```python
from build123d import *

# Parameters (mm, degrees)
F0_W     = 38.1
F0_H     = 38.1
F0_W_2   = 31.75
F0_H_2   = 31.75
F1_DEPTH = 2743.2
F2_R     = 6.35
F3_DEPTH = 38.101


# Not quite as in the source:
# - a feature names something its author has since deleted; it is built from what else it names


with BuildPart() as f1:
    # F0 (on Front) → F1 (new body)
    with BuildSketch(Plane.XZ):
        Rectangle(F0_W, F0_H)
        Rectangle(F0_W_2, F0_H_2, mode=Mode.SUBTRACT)
    extrude(amount=F1_DEPTH)

    # F2 (on face) → F3 (cut, through all)
    with BuildSketch(Plane.XY.offset(19.05)):
        with Locations((0, -25.4)):
            Circle(F2_R)
        with Locations((0, -76.2)):
            Circle(F2_R)
        with Locations((0, -2717.8)):
            Circle(F2_R)
        with Locations((0, -2667)):
            Circle(F2_R)
    extrude(amount=-F3_DEPTH, mode=Mode.SUBTRACT)


solid = f1.part
```
Check sheet for the modelled part. Datum: model origin and axes. Units: mm. Round coordinates to 2 decimals unless told otherwise and drop trailing zeros. Loops run counter-clockwise (first coordinate to the right, second up) from the corner with the lowest first, then second, coordinate; pieces in that order, holes last. Notation, with made-up numbers: (24.5, 19.25) -> (63.5, 19.25) arc R18 ccw to (63.5, 51.25) -> close; hole circle Ø2 at (75.25, -27.5). An arc over 180 degrees is marked (long way). Answer in a Markdown table with one row per item.
Q1. Sectioned sample at A-A on z = 6. Enter the section's corners in (x, y) (3 decimals), then the cut area to 3 significant figures.
Data:
| item | result |
|---|---|
| outline | (-19.05, -2743.2) -> (-15.875, -2743.2) -> (-15.875, 0) -> (-19.05, 0) -> close; (15.875, -2743.2) -> (19.05, -2743.2) -> (19.05, 0) -> (15.875, 0) -> close |
| area | 17,400 mm^2 |
Q2. Sectioned sample at C-C on x = 0. Give the number of separate pieces and of enclosed holes in the cut face, then the cut area to 3 significant figures.
Data:
| item | result |
|---|---|
| separate pieces | 10 |
| enclosed holes | 0 |
| area | 17,100 mm^2 |
Q3. Go/stop test with a flat-tipped pin: P1, Ø8, axis at x = 12.5, z = 14, coming from the -Y side. Record where the tip stops, or that it passes through.
Data:
| item | result |
|---|---|
| P1 | stops at y = -2743.2 |
Q4. Sectioned sample at B-B on y = -1659.5. Enter the section's corners in (x, z) (3 decimals).
Data:
| item | result |
|---|---|
| outline | (-19.05, -19.05) -> (19.05, -19.05) -> (19.05, 19.05) -> (-19.05, 19.05) -> close; hole (-15.875, -15.875) -> (15.875, -15.875) -> (15.875, 15.875) -> (-15.875, 15.875) -> close |
Q5. Thickness scan on L1, parallel to Y at x = 0, z = 16.65; L2, parallel to X at y = -2717, z = -17; L3, parallel to Z at x = -12.5, y = -1379.5 (3 decimals). Record the ranges inside material, lowest first.
Data:
| item | result |
|---|---|
| L1 | y = -2743.2 to -2724.15, -2711.45 to -2673.35, -2660.65 to -82.55, -69.85 to -31.75, -19.05 to 0 |
| L2 | x = -19.05 to -6.3, 6.3 to 19.05 |
| L3 | z = -19.05 to -15.875, 15.875 to 19.05 |
